Print and shaded views of the part. All mm, measured from the part's lowest x, y and z. A direction names the side the tool comes from. Round coordinates to 2 decimals unless told otherwise and drop trailing zeros. Write each loop counter-clockwise with the first axis right and the second up, starting at its lowest first coordinate (ties: lowest second). Pieces come first, ordered by that corner, then holes. Notation, with made-up numbers: (39.25, 72) - (93.25, 72) arc R16 ccw to (93.25, 85) - close; hole circle Ø3 at (18.5, -26.75). An arc over 180 degrees is marked (long way). Put each result on its own line as item: value. Start each with the question number.
Item 1: 3-axis set-ups, long thin cutter, end or side, ignore diameter. For the marked faces 5, 6 and 7: which of +Z, -Z, +X, -X, +Y, -Y reach the whole face in a straight line?
Item 2: Cut at D-D (z = 19.25). Give the cut face in (x, y).
Item 3: Drill centre lines: line 1 (X direction, y = 6, z = 18.5); line 2 (Z direction, x = 0.75, y = 6); line 3 (X direction, y = 6, z = 9.75). Where is each one in solid material? Low to high. Write a range as from..to.
Item 4: Mould opens along X. For the marked faces 1, 2, 3 and 4 say: released by +X, released by -X, zero draft, split by the parting line, or undercut.
Item 5: Cut at A-A (y = 6). Give the cut face in (x, z), and give its area (3 significant figures).
Item 6: Pin check, flat tips, straight feed: pin 1 Ø3.5 at (y, z) = (6, 14) entering from -X; pin 2 Ø2.5 at (x, y) = (7, 6) entering from -Z; pin 3 Ø4.5 at (x, y) = (6, 6) entering from +Z. Stop position of each tip, or through.
Item 7: Cut at B-B (z = 14.5). Give the cut face in (x, y), and give its area (3 significant figures).
Item 8: Cut at C-C (x = 6). Give the cut face in (y, z), and give its area (3 significant figures).
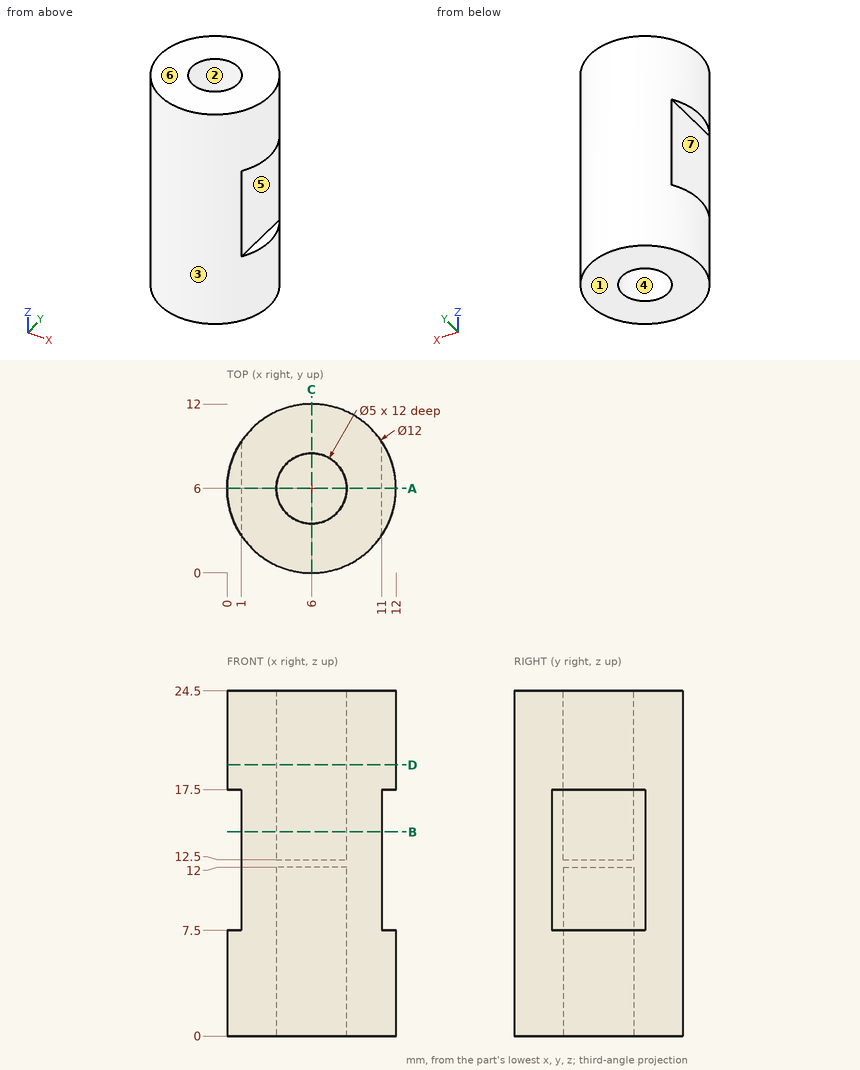
Output values:
1. face 5: +X, +Y, -Y
1. face 6: +Z, +X, -X, +Y, -Y
1. face 7: -X, +Y, -Y
2. outline: circle Ø12 at (6, 6); hole circle Ø5 at (6, 6)
3. line 1: 0..3.5, 8.5..12
3. line 2: 0..7.5, 17.5..24.5
3. line 3: 1..3.5, 8.5..11
4. face 1: zero draft
4. face 2: undercut
4. face 3: split by the parting line
4. face 4: undercut
5. outline: (0, 0) - (3.5, 0) - (3.5, 12) - (8.5, 12) - (8.5, 0) - (12, 0) - (12, 7.5) - (11, 7.5) - (11, 17.5) - (12, 17.5) - (12, 24.5) - (8.5, 24.5) - (8.5, 12.5) - (3.5, 12.5) - (3.5, 24.5) - (0, 24.5) - (0, 17.5) - (1, 17.5) - (1, 7.5) - (0, 7.5) - close
5. area: 154 mm2
6. pin 1: x = 1
6. pin 2: z = 12
6. pin 3: z = 12.5
7. outline: (1, 2.68) arc R6 ccw to (11, 2.68) - (11, 9.32) arc R6 ccw to (1, 9.32) - close; hole circle Ø5 at (6, 6)
7. area: 84.5 mm2
8. outline: (0, 0) - (3.5, 0) - (3.5, 12) - (8.5, 12) - (8.5, 0) - (12, 0) - (12, 24.5) - (8.5, 24.5) - (8.5, 12.5) - (3.5, 12.5) - (3.5, 24.5) - (0, 24.5) - close
8. area: 174 mm2
